The listing builds one solid part. Answer for the finished solid, in the listing's coordinates (mm). A direction names the side the tool comes from. Coordinates: 2 decimals unless noted, no trailing zeros. Order: outer loops, then holes, each group sorted by start corner. A loop starts at its lowest first (then second) coordinate and runs counter-clockwise, first axis right, second up. Notation, with made-up numbers: (54, 58.25) - (105, 58.25) arc R22 ccw to (105, 95.25) - close; hole circle Ø8 at (20, -23). An arc over 180 degrees is marked (long way). Use a Markdown table: item, result. Add a question column.
Item 1: The part is cut by section D-D, the plane y = -40. Give the vertices of the cut face in (x, z).
Item 2: For faces 1 (the cylindrical face through (-121.74, -50.09, -91.68)), 2 (the flat face through (-63.88, -88.722, -39.553)), determine the directions among +Z, -Z, +X, -X, +Y, -Y from which every point of the face is accessible in a straight line to the end or side of a thin tool.
Item 3: The part is cut by section C-C, the plane z = -25.5. Give the vertices of the cut face in (x, y), then the cut area to 3 significant figures.
Item 4: Flat-ended cylindrical pins translate along their axes: P1, Ø5, axis at y = -62, z = -83.5, coming from the +X side; P2, Ø8, axis at y = -12.5, z = -12, coming from the +X side; P3, Ø8, axis at x = -74, y = -91, coming from the -Z side. Find the tip coordinate at first contact, or state that the pin passes through.
Item 5: The part is cut by section B-B, the plane x = -96. Give the vertices of the cut face in (y, z), then the cut area to 3 significant figures.
Item 6: Find the intervals of material crossed by line 1 along Y through (x, z) = (-114, -18.5); line 2 along Y through (x, z) = (-64.5, -36.5); line 3 along Z through (x, y) = (-72.5, -28), in increasing order.
Item 7: The part is cut by section A-A, the plane y = -22.5. Give the vertices of the cut face in (x, z).
from build123d import *

# Parameters (mm, degrees)
F1_DEPTH = 25.4
F2_DEPTH = 50.8
F3_DEPTH = 76.2
F4_DEPTH = 101.6


with BuildPart() as f1:
    # F0 (on Front) → F1 (new body)
    with BuildSketch(Plane.XZ):
        with BuildLine():
            Line((0, 0), (-152.4, 0))
            ThreePointArc((-152.4, 0), (-151.749888, -14.061698), (-149.8051, -28.003427))
            Line((-149.8051, -28.003427), (0, 0))
        make_face()
    extrude(amount=F1_DEPTH)

    # F0 (on Front) → F2 (join)
    with BuildSketch(Plane.XZ):
        with BuildLine():
            Line((-142.108768, -55.05323), (0, 0))
            Line((0, 0), (-149.8051, -28.003427))
            ThreePointArc((-149.8051, -28.003427), (-146.582228, -41.70624), (-142.108768, -55.05323))
        make_face()
    extrude(amount=F2_DEPTH)

    # F0 (on Front) → F3 (join)
    with BuildSketch(Plane.XZ):
        with BuildLine():
            Line((-129.573091, -80.228262), (0, 0))
            Line((0, 0), (-142.108768, -55.05323))
            ThreePointArc((-142.108768, -55.05323), (-136.422886, -67.930525), (-129.573091, -80.228262))
        make_face()
    extrude(amount=F3_DEPTH)

    # F0 (on Front) → F4 (join)
    with BuildSketch(Plane.XZ):
        with BuildLine():
            Line((-112.624959, -102.671216), (0, 0))
            Line((0, 0), (-129.573091, -80.228262))
            ThreePointArc((-129.573091, -80.228262), (-121.617825, -91.841519), (-112.624959, -102.671216))
        make_face()
    extrude(amount=F4_DEPTH)


solid = f1.part
Solution:
| question | item | result |
|---|---|---|
| 1 | outline | (-149.81, -28) arc R152.4 ccw to (-142.11, -55.05) arc R152.4 ccw to (-129.57, -80.23) arc R152.4 ccw to (-112.62, -102.67) - (0, 0) - close |
| 2 | face 1 | -Z, -X, +Y, -Y |
| 2 | face 2 | +Z, -X, -Y |
| 3 | outline | (-150.25, -25.4) - (-136.41, -25.4) - (-136.41, -50.8) - (-65.82, -50.8) - (-65.82, -76.2) - (-41.18, -76.2) - (-41.18, -101.6) - (-27.97, -101.6) - (-27.97, 0) - (-150.25, 0) - close |
| 3 | area | 7,160 mm2 |
| 4 | P1 | stops at x = -88.85 |
| 4 | P2 | stops at x = -8.78 |
| 4 | P3 | stops at z = -71.11 |
| 5 | outline | (-101.6, -87.52) - (0, -87.52) - (0, 0) - (-25.4, 0) - (-25.4, -17.95) - (-50.8, -17.95) - (-50.8, -37.19) - (-76.2, -37.19) - (-76.2, -59.44) - (-101.6, -59.44) - close |
| 5 | area | 5,980 mm2 |
| 6 | line 1 | y = -25.4 to 0 |
| 6 | line 2 | y = -76.2 to 0 |
| 6 | line 3 | z = -66.09 to -13.55 |
| 7 | outline | (-152.4, 0) arc R152.4 ccw to (-149.81, -28) arc R152.4 ccw to (-142.11, -55.05) arc R152.4 ccw to (-129.57, -80.23) arc R152.4 ccw to (-112.62, -102.67) - (0, 0) - close |
